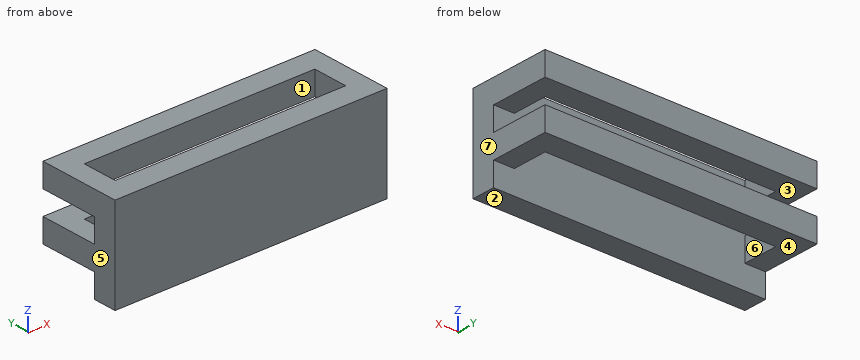
```python
from build123d import *

# Parameters (mm, degrees)
F0_W     = 23.068964
F0_H     = 7
F0_W_2   = 19.551722
F0_H_2   = 3
F1_DEPTH = 2
F3_DEPTH = 2
F5_DEPTH = 2
F7_DEPTH = 2


with BuildPart() as f1:
    # F0 (on Top) → F1 (new body)
    with BuildSketch(Plane.XY):
        with Locations((2.640947, 3.5)):
            Rectangle(F0_W, F0_H)
        with Locations((2.640947, 3.5)):
            Rectangle(F0_W_2, F0_H_2, mode=Mode.SUBTRACT)
    extrude(amount=F1_DEPTH)

    # F2 (on face) → F3 (join)
    with BuildSketch(Plane(origin=(0, 0, 0), x_dir=(1, 0, 0), z_dir=(0, 0, -1))):
        Polygon((14.175429, -2), (14.175429, 0), (-8.893535, 0), (-8.893535, -2), (-7.134914, -2), (12.416808, -2), align=None)
    extrude(amount=F3_DEPTH)

    # F4 (on face) → F5 (join)
    with BuildSketch(Plane.XY.offset(2)):
        Polygon((-8.893535, 2), (-8.893535, 0), (14.175429, 0), (14.175429, 2), (12.416808, 2), (-7.134914, 2), align=None)
    extrude(amount=F5_DEPTH)

    # F6 (on face) → F7 (join)
    with BuildSketch(Plane.XY.offset(4)):
        Polygon((-7.134914, 2), (-8.893535, 2), (-8.893535, 0), (14.175429, 0), (14.175429, 2), (12.416808, 2), align=None)
        Polygon((-8.893535, 7), (-8.893535, 2), (-7.134914, 2), (-7.134914, 5), (12.416808, 5), (12.416808, 2), (14.175429, 2), (14.175429, 7), align=None)
    extrude(amount=F7_DEPTH)


solid = f1.part
```
Source: CAD feature listing. Evaluate the final solid. Frame: model axes, mm. Face numbers are marked on the shaded views. A direction names the side the tool comes from. Round coordinates to 2 decimals unless told otherwise and drop trailing zeros. Loops run counter-clockwise (first coordinate to the right, second up) from the corner with the lowest first, then second, coordinate; pieces in that order, holes last.
(1) Material intervals for probe 1 along Y at (x, z) = (0, 1.25); probe 2 along Z at (x, y) = (2, 5.75); probe 3 along X at (y, z) = (4.5, 1.25), sorted ascending.
From the geometry:
probe 1: y = 0 to 2, 5 to 7
probe 2: z = 0 to 2, 4 to 6
probe 3: x = -8.89 to -7.13, 12.42 to 14.18
(2) Access query for the marked faces 1, 2 and 3. Directions: +Z, -Z, +X, -X, +Y, -Y. A direction counts if a zero-diameter tool reaches every point of the face in a straight line with its end or side. Return the directions, or none.
From the geometry:
face 1: +Z, -Z
face 2: -Z, +X, -X, +Y, -Y
face 3: +X, -X, +Y
(3) Section query D-D (y = 3.5). Output: boundary loops of the cut face in (x, z).
From the geometry:
outline: (-8.89, 0) - (-7.13, 0) - (-7.13, 2) - (-8.89, 2) - close; (-8.89, 4) - (-7.13, 4) - (-7.13, 6) - (-8.89, 6) - close; (12.42, 0) - (14.18, 0) - (14.18, 2) - (12.42, 2) - close; (12.42, 4) - (14.18, 4) - (14.18, 6) - (12.42, 6) - close
(4) Section query C-C (x = -4). Output: boundary loops of the cut face in (y, z), and give its area (3 significant figures).
From the geometry:
outline: (0, -2) - (2, -2) - (2, 6) - (0, 6) - close; (5, 0) - (7, 0) - (7, 2) - (5, 2) - close; (5, 4) - (7, 4) - (7, 6) - (5, 6) - close
area: 24.0 mm2
(5) Pull-direction query (X, two-part tool) for the marked faces 4, 5, 6 and 7; classes: +X half, -X half, draft (parallel to the pull), parting line (faces both ways), or undercut.
From the geometry:
face 4: draft
face 5: -X half
face 6: undercut
face 7: +X half
(6) Section query A-A (z = 4.5). Output: boundary loops of the cut face in (x, y), and give its area (3 significant figures).
From the geometry:
outline: (-8.89, 0) - (14.18, 0) - (14.18, 7) - (-8.89, 7) - close; hole (-7.13, 2) - (12.42, 2) - (12.42, 5) - (-7.13, 5) - close
area: 103 mm2
(7) Section query B-B (y = 5.25). Output: boundary loops of the cut face in (x, z).
From the geometry:
outline: (-8.89, 0) - (14.18, 0) - (14.18, 2) - (-8.89, 2) - close; (-8.89, 4) - (14.18, 4) - (14.18, 6) - (-8.89, 6) - close
(8) Contact query for flat-ended pins moving along their axis: pin 1 Ø1.6 at (x, z) = (2, 1) entering from -Y; pin 2 Ø1.5 at (x, y) = (7, 4) entering from -Z. Output: stop coordinate, or through.
From the geometry:
pin 1: stops at y = 0
pin 2: passes through
